Here's the drawing with two shaded views (mm, measured from the low corner). I have some questions. A direction names the side the tool comes from. Coordinates: 2 decimals unless noted, no trailing zeros. Write each loop counter-clockwise with the first axis right and the second up, starting at its lowest first coordinate (ties: lowest second). Pieces come first, ordered by that corner, then holes.
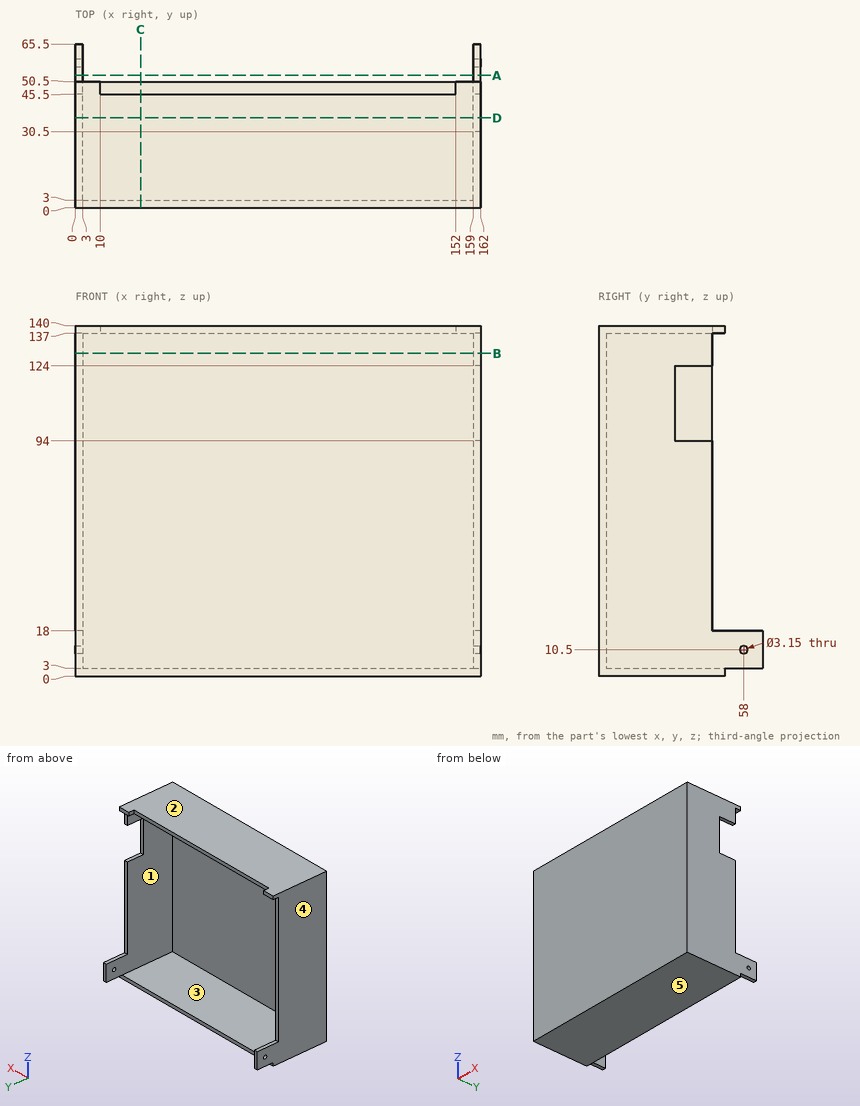
Item 1: If we mould it in two halves opening along X, with no side actions, what happens to the marked faces 3, 4 and 5? For each: released by +X, released by -X, zero draft, split by the parting line, or undercut.
Item 2: I want a section at D-D, the plane y = 36. List the corners of the cut face in (x, z) for me, then the cut area to 3 significant figures.
Item 3: I want a section at A-A, the plane y = 53. List the corners of the cut face in (x, z) for me, then the cut area to 3 significant figures.
Item 4: I want a section at C-C, the plane x = 26. List the corners of the cut face in (y, z) for me.
Item 5: Which directions (+Z, -Z, +X, -X, +Y, -Y) give clear straight access to the entire face, cutting with the end or side of a thin tool? Please do the marked faces 1 and 2.
Item 6: If I drill on line 1 along Z through (x, y) = (57.5, 12); line 2 along Y through (x, z) = (2.15, 10.5) (3 decimals); line 3 along X through (y, z) = (32, 44.5), over which ranges is the centre line in solid material (lowest first)?
Item 7: I want a section at B-B, the plane z = 129. List the corners of the cut face in (x, y) for me.
Item 8: Will these pins go through, and if not, where does the flat tip stop? pin 1 Ø1.5 at (x, y) = (1.5, 59.5) entering from -Z; pin 2 Ø1.9 at (y, z) = (58, 10.5) entering from -X; pin 3 Ø2 at (x, y) = (117.5, 48.5) entering from +Z; pin 4 Ø2.5 at (x, z) = (59, 138) entering from +Y.
Taken from the geometry:
1. face 3: undercut
1. face 4: released by -X
1. face 5: zero draft
2. outline: (0, 0) - (162, 0) - (162, 94) - (159, 94) - (159, 3) - (3, 3) - (3, 137) - (159, 137) - (159, 124) - (162, 124) - (162, 140) - (0, 140) - close
2. area: 1,690 mm2
3. outline: (0, 3) - (3, 3) - (3, 18) - (0, 18) - close; (159, 3) - (162, 3) - (162, 18) - (159, 18) - close
3. area: 90.0 mm2
4. outline: (0, 0) - (50.5, 0) - (50.5, 3) - (3, 3) - (3, 137) - (45.5, 137) - (45.5, 140) - (0, 140) - close
5. face 1: +Y
5. face 2: +Z, +X, -X, +Y, -Y
6. line 1: z = 0 to 3, 137 to 140
6. line 2: y = 0 to 56.425, 59.575 to 65.5
6. line 3: x = 0 to 3, 159 to 162
7. outline: (0, 0) - (162, 0) - (162, 45.5) - (159, 45.5) - (159, 3) - (3, 3) - (3, 45.5) - (0, 45.5) - close
8. pin 1: stops at z = 3
8. pin 2: passes through
8. pin 3: stops at z = 3
8. pin 4: stops at y = 45.5
